CAD build for the part. Positions are in the model's coordinates, mm. Coordinates: 2 decimals unless noted, no trailing zeros. Order: outer loops, then holes, each group sorted by start corner. A loop starts at its lowest first (then second) coordinate and runs counter-clockwise, first axis right, second up.
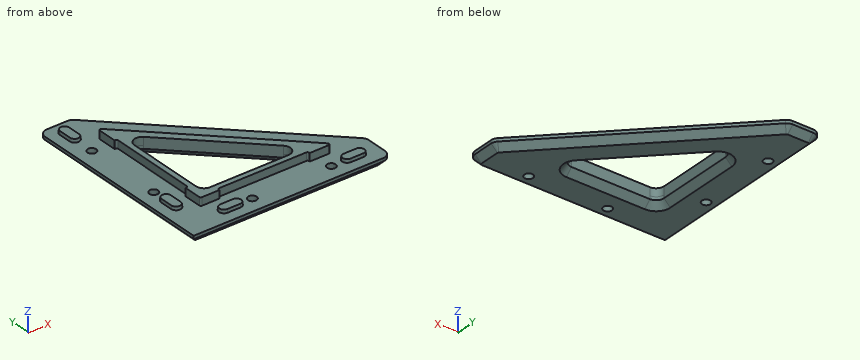
from build123d import *

# Parameters (mm, degrees)
F1_DEPTH  = 6
F2_R      = 5
F4_DEPTH  = 5
F5_SIZE   = 4
F6_R      = 1
F8_D      = 5.5
F9_W      = 57.1730165467
F9_H      = 1.5
F9_W_2    = 1.5
F9_H_2    = 57.372583002
F10_DEPTH = 5
F11_R     = 1
F13_DEPTH = 2
F13_TAPER = 8


with BuildPart() as f1:
    # F0 (on Top) → F1 (new body)
    with BuildSketch(Plane.XY):
        Polygon((20, 125), (0, 125), (0, 0), (125, 0), (125, 20), align=None)
        Polygon((25, 25), (25, 91.7157287525), (91.7157287525, 25), align=None, mode=Mode.SUBTRACT)
    extrude(amount=F1_DEPTH)

    # F2
    f2_edges = [f1.edges().sort_by_distance(p)[0] for p in [
        (25, 91.715729, 3),
        (91.715729, 25, 3),
        (25, 25, 3),
        (0, 125, 3),
        (20, 125, 3),
        (125, 20, 3),
        (125, 0, 3),
    ]]
    fillet(f2_edges, radius=F2_R)

    # F3 (on face) → F4 (join)
    with BuildSketch(Plane.XY.offset(6)):
        Polygon((86.7157287525, 37.0710678119), (37.0710678119, 86.7157287525), (20, 103.7867965644), (20, 79.6446609407), (20, 30), (20, 20), (30, 20), (79.6446609407, 20), (103.5650894046, 20), align=None)
        with BuildLine():
            ThreePointArc((30, 25), (26.4644660941, 26.4644660941), (25, 30))
            Line((25, 30), (25, 79.6446609407))
            ThreePointArc((25, 79.6446609407), (28.0865828382, 84.2640586032), (33.5355339059, 83.1801948466))
            Line((33.5355339059, 83.1801948466), (83.1801948466, 33.5355339059))
            ThreePointArc((83.1801948466, 33.5355339059), (84.2640586032, 28.0865828382), (79.6446609407, 25))
            Line((79.6446609407, 25), (30, 25))
        make_face(mode=Mode.SUBTRACT)
    extrude(amount=F4_DEPTH)

    # F5
    f5_edges = [f1.edges().sort_by_distance(p)[0] for p in [
        (58.357864, 58.357864, 0),
        (72.5, 72.5, 0),
    ]]
    chamfer(f5_edges, length=F5_SIZE)

    # F6
    f6_edges = [f1.edges().sort_by_distance(p)[0] for p in [
        (20, 103.786797, 8.5),
        (20, 20, 8.5),
        (103.565089, 20, 8.5),
    ]]
    fillet(f6_edges, radius=F6_R)

    # F8 (through all)
    with Locations(Plane(origin=(0, 0, 0), x_dir=(1, 0, 0), z_dir=(0, 0, -1))):
        with Locations((95, -10), (45, -10), (10, -45), (10, -95)):
            Hole(F8_D / 2)

    # F9 (on face) → F10 (cut, through all)
    with BuildSketch(Plane.XY.offset(11)):
        with Locations((60.5865082733, 20.75)):
            Rectangle(F9_W, F9_H)
        with Locations((20.75, 60.686291501)):
            Rectangle(F9_W_2, F9_H_2)
    extrude(amount=-F10_DEPTH, mode=Mode.SUBTRACT)

    # F11
    f11_edges = [f1.edges().sort_by_distance(p)[0] for p in [
        (21.5, 89.372583, 8.5),
        (21.5, 32, 8.5),
        (32, 21.5, 8.5),
        (89.173017, 21.5, 8.5),
    ]]
    fillet(f11_edges, radius=F11_R)

    # F12 (on face) → F13 (join)
    with BuildSketch(Plane.XY.offset(6)):
        with BuildLine():
            Line((6.85, 117), (6.85, 109))
            ThreePointArc((6.85, 109), (10, 105.85), (13.15, 109))
            Line((13.15, 109), (13.15, 117))
            ThreePointArc((13.15, 117), (10, 120.15), (6.85, 117))
        make_face()
        with BuildLine():
            Line((6.85, 35), (6.85, 27))
            ThreePointArc((6.85, 27), (10, 23.85), (13.15, 27))
            Line((13.15, 27), (13.15, 35))
            ThreePointArc((13.15, 35), (10, 38.15), (6.85, 35))
        make_face()
        with BuildLine():
            Line((35, 13.15), (27, 13.15))
            ThreePointArc((27, 13.15), (23.85, 10), (27, 6.85))
            Line((27, 6.85), (35, 6.85))
            ThreePointArc((35, 6.85), (38.15, 10), (35, 13.15))
        make_face()
        with BuildLine():
            Line((113, 13.15), (105, 13.15))
            ThreePointArc((105, 13.15), (101.85, 10), (105, 6.85))
            Line((105, 6.85), (113, 6.85))
            ThreePointArc((113, 6.85), (116.15, 10), (113, 13.15))
        make_face()
    extrude(amount=F13_DEPTH, taper=F13_TAPER)


solid = f1.part
1) Slice it at A-A (x = 10). List the corners of the cut face in (y, z).
2) Drill centre lines: probe 1 along Y at (x, z) = (10, 4.7); probe 2 along X at (y, z) = (45, 2.85). Where is each one in solid material? Low to high.
3) Pin check, flat tips, straight feed: P1, Ø6.5, axis at x = 108.5, y = 11, coming from the +Z side; P2, Ø10, axis at x = 29, y = 70.5, coming from the -Z side; P3, Ø2, axis at x = 42.5, z = 6.5, coming from the +Y side; P4, Ø3.5, axis at x = 10, y = 95, coming from the +Z side. Stop position of each tip, or through.
4) Slice it at C-C (y = 95). List the corners of the cut face in (x, z), plus the area to 3 significant figures.
5) Slice it at D-D (x = 95). List the corners of the cut face in (y, z), plus the area to 3 significant figures.
6) Slice it at B-B (y = 10). List the corners of the cut face in (x, z).
Worked out:
1. outline: (0, 4) - (4, 0) - (42.25, 0) - (42.25, 6) - (38.15, 6) - (37.87, 8) - (24.13, 8) - (23.85, 6) - (0, 6) - close; (47.75, 0) - (92.25, 0) - (92.25, 6) - (47.75, 6) - close; (97.75, 0) - (121, 0) - (125, 4) - (125, 6) - (120.15, 6) - (119.87, 8) - (106.13, 8) - (105.85, 6) - (97.75, 6) - close
2. probe 1: y = 0 to 42.25, 47.75 to 92.25, 97.75 to 125
2. probe 2: x = 1.15 to 7.25, 12.75 to 23.85, 73.34 to 98.37
3. P1: stops at z = 8
3. P2: stops at z = 3
3. P3: stops at y = 103.37
3. P4: passes through
4. outline: (0, 4) - (4, 0) - (7.25, 0) - (7.25, 6) - (0, 6) - close; (12.75, 0) - (44.34, 0) - (50, 4) - (50, 6) - (28.79, 6) - (28.79, 11) - (20, 11) - (20, 6) - (12.75, 6) - close
4. area: 292 mm2
5. outline: (0, 4) - (4, 0) - (7.25, 0) - (7.25, 6) - (0, 6) - close; (12.75, 0) - (44.34, 0) - (50, 4) - (50, 6) - (28.68, 6) - (28.68, 11) - (20, 11) - (20, 6) - (12.75, 6) - close
5. area: 291 mm2
6. outline: (0, 4) - (4, 0) - (42.25, 0) - (42.25, 6) - (38.15, 6) - (37.87, 8) - (24.13, 8) - (23.85, 6) - (0, 6) - close; (47.75, 0) - (92.25, 0) - (92.25, 6) - (47.75, 6) - close; (97.75, 0) - (121, 0) - (125, 4) - (125, 6) - (116.15, 6) - (115.87, 8) - (102.13, 8) - (101.85, 6) - (97.75, 6) - close
